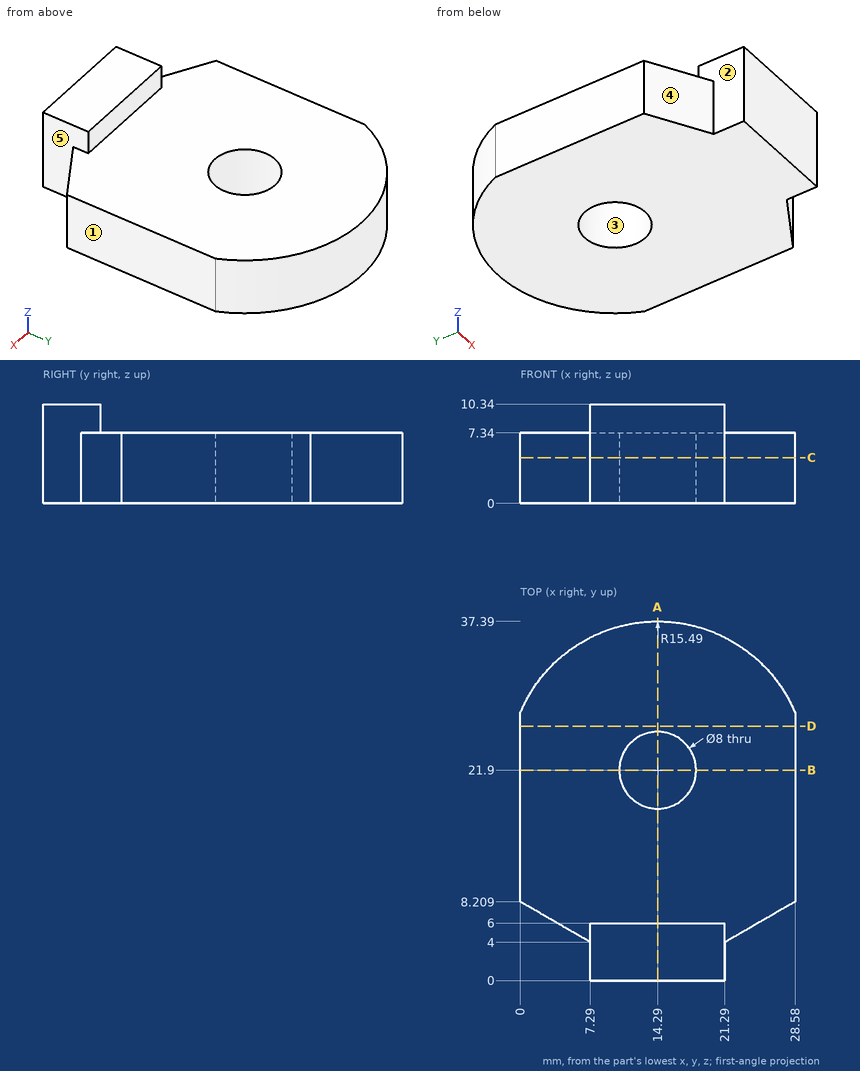
Study the drawing (mm; zero at the part's minimum x, y, z) and answer. A direction names the side the tool comes from. Give positions to 0.01 mm unless a question says otherwise; leave off trailing zeros. Order: outer loops, then holes, each group sorted by start corner. A loop starts at its lowest first (then second) coordinate and runs counter-clockwise, first axis right, second up. Notation, with made-up numbers: (-3.5, 39) -> (31.5, 39) arc R26 ccw to (31.5, 74) -> close; hole circle Ø1 at (38.5, 82). An arc over 180 degrees is marked (long way). Put each result on its own line as item: value.
Item 1: A cutting plane is placed at B-B on y = 21.9. Give the vertices of the cut face in (x, z), plus the area to 3 significant figures.
Established:
outline: (0, 0) -> (10.29, 0) -> (10.29, 7.34) -> (0, 7.34) -> close; (18.29, 0) -> (28.58, 0) -> (28.58, 7.34) -> (18.29, 7.34) -> close
area: 151 mm^2
Item 2: A cutting plane is placed at C-C on z = 4.75. Give the vertices of the cut face in (x, y), plus the area to 3 significant figures.
Established:
outline: (0, 8.21) -> (7.29, 4) -> (7.29, 0) -> (21.29, 0) -> (21.29, 4) -> (28.58, 8.21) -> (28.58, 27.88) arc R15.49 ccw to (0, 27.88) -> close; hole circle Ø8 at (14.29, 21.9)
area: 854 mm^2
Item 3: Given P1, Ø8.5, axis at x = 11.5, y = 14.5, coming from the +Z side; P2, Ø0.9, axis at x = 15.5, z = 8.5, coming from the +Y side; P3, Ø1.8, axis at y = 3, z = 4, coming from the +X side; P4, Ø6, axis at x = 7.5, y = 23.5, coming from the -Z side, each flat-ended and moving along its own axis, determine where each tip first touches the part or whether it passes through.
Established:
P1: stops at z = 7.34
P2: stops at y = 6
P3: stops at x = 21.29
P4: stops at z = 0
Item 4: A cutting plane is placed at A-A on x = 14.29. Give the vertices of the cut face in (y, z), plus the area to 3 significant figures.
Established:
outline: (0, 0) -> (17.9, 0) -> (17.9, 7.34) -> (6, 7.34) -> (6, 10.34) -> (0, 10.34) -> close; (25.9, 0) -> (37.39, 0) -> (37.39, 7.34) -> (25.9, 7.34) -> close
area: 234 mm^2
Item 5: For the marked faces 1 and 2, determine the directions among +Z, -Z, +X, -X, +Y, -Y from which every point of the face is accessible in a straight line to the end or side of a thin tool.
Established:
face 1: +Z, -Z, +X, +Y, -Y
face 2: +Z, -X, -Y
Item 6: Straight lines are drawn through the part: line 1 (Y direction, x = 14.29, z = 4.25); line 2 (Z direction, x = 4.5, y = 17.5); line 3 (Y direction, x = 18.75, z = 7.5). For each, find the intervals that lie inside material, in ascending order.
Established:
line 1: y = 0 to 17.9, 25.9 to 37.39
line 2: z = 0 to 7.34
line 3: y = 0 to 6
Item 7: For a pull along Y with two mould halves and no side action, classify the marked faces 3, 4 and 5 as released by +Y, released by -Y, zero draft, split by the parting line, or undercut.
Established:
face 3: undercut
face 4: released by -Y
face 5: zero draft
Item 8: A cutting plane is placed at D-D on y = 26.5. Give the vertices of the cut face in (x, z), plus the area to 3 significant figures.
Established:
outline: (0, 0) -> (28.58, 0) -> (28.58, 7.34) -> (0, 7.34) -> close
area: 210 mm^2
